from build123d import *

# Parameters (mm, degrees)
F0_W     = 76.2
F0_H     = 76.2
F1_DEPTH = 101.6
F3_DEPTH = 101.6


with BuildPart() as f1:
    # F0 (on Right) → F1 (new body)
    with BuildSketch(Plane.YZ):
        with Locations((38.1, 38.1)):
            Rectangle(F0_W, F0_H)
    extrude(amount=F1_DEPTH)

    # F2 (on face) → F3 (join)
    with BuildSketch(Plane.YZ.offset(101.6)):
        Polygon((-27.540024, 26.327876), (-36.570622, -10.686423), (-9.030597, -37.014299), (27.540024, -26.327876), (33.963392, 0), (0, 0), (0, 34.375438), align=None)
        Polygon((9.030597, 37.014299), (0, 34.375438), (0, 0), (33.963392, 0), (36.570622, 10.686423), align=None)
    extrude(amount=F3_DEPTH)


solid = f1.part
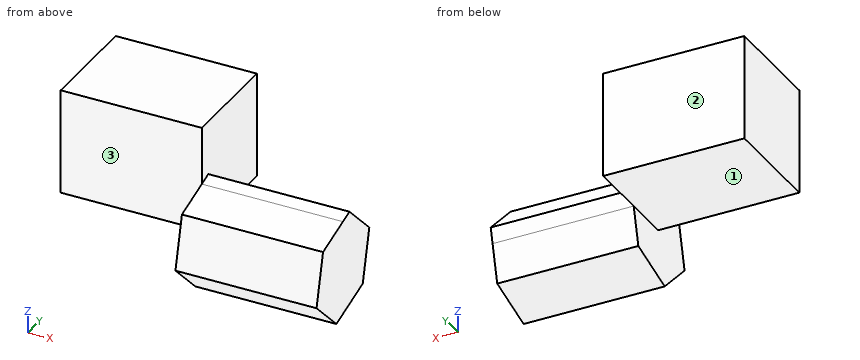
Model file for the job. Use its own axes, mm. Face numbers are marked on the shaded views. A direction names the side the tool comes from. Coordinates: 2 decimals unless noted, no trailing zeros. Order: outer loops, then holes, each group sorted by start corner. A loop starts at its lowest first (then second) coordinate and runs counter-clockwise, first axis right, second up. Notation, with made-up numbers: (52, -21) -> (75, -21) arc R28 ccw to (75, 16) -> close; hole circle Ø5 at (45, -7). An arc over 180 degrees is marked (long way). Return JSON: item names as keys, results as strings. Group by question number.
Item 1: Saw through at A-A on x = 115. Write the cut outline in (y, z), then the cut area to 3 significant figures.
Item 2: Flat gauge pins, fed straight in: P1, Ø3, axis at x = 152, z = 1.5, coming from the -Y side; P2, Ø4, axis at x = 98, z = 33, coming from the -Y side; P3, Ø8, axis at x = 85, y = 21, coming from the -Z side. Where does each tip first touch, or does it go through?
Item 3: Saw through at C-C on z = 69. Write the cut outline in (x, y).
Item 4: Tool access for the marked faces 1, 2 and 3: list every direction of +Z, -Z, +X, -X, +Y, -Y with a clear straight run to the whole face (end or side of a thin tool).
Item 5: Saw through at B-B on y = 31. Write the cut outline in (x, z), then the cut area to 3 significant figures.
Item 6: Wall check: line 1 along X through (y, z) = (71, 42); line 2 along X through (y, z) = (7.5, -13); line 3 along Y through (x, z) = (66, 45). Give the ranges that are in metal, low to high. Write a range as [from, to].
Values found:
{
 "1": {"outline": "(-36.57, -10.69) -> (-9.03, -37.01) -> (27.54, -26.33) -> (36.57, 10.69) -> (9.03, 37.01) -> (-27.54, 26.33) -> close", "area": "3,770 mm2"},
 "2": {"P1": "stops at y = -33.96", "P2": "stops at y = 0", "P3": "stops at z = 0"},
 "3": {"outline": "(0, 0) -> (101.6, 0) -> (101.6, 76.2) -> (0, 76.2) -> close"},
 "4": {"face 1": "-Z, -X, +Y, -Y", "face 2": "+Z, -Z, +X, -X, +Y", "face 3": "+Z, -Z, -X, -Y"},
 "5": {"outline": "(0, 0) -> (101.6, 0) -> (101.6, -12.15) -> (203.2, -12.15) -> (203.2, 16.01) -> (101.6, 16.01) -> (101.6, 76.2) -> (0, 76.2) -> close", "area": "10,600 mm2"},
 "6": {"line 1": "x = [0, 101.6]", "line 2": "x = [101.6, 203.2]", "line 3": "y = [0, 76.2]"}
}
